Can you work these out from the model? Positions are in its coordinate system, mm. A direction names the side the tool comes from. Give positions to 0.01 mm unless a question says otherwise; leave off trailing zeros. Order: outer loops, then holes, each group sorted by start corner. A loop starts at its lowest first (then second) coordinate and runs counter-clockwise, first axis right, second up. Notation, with made-up numbers: (12, 10.5) -> (54, 10.5) arc R28 cw to (54, 36.5) -> close; hole circle Ø6 at (17, 40.25). An arc over 180 degrees is marked (long way). Answer as a JSON object with one key per item and string values.
Solid Edge part; units mm, degrees
sketch "Sketch1" plane through (0, 0, 0) normal (0, -1, 0) x (1, 0, 0)
  line L0 (0, 19.05) -> (0, 0)
  line L1 (0, 0) -> (19.05, 0)
  line L2 (19.05, 0) -> (19.05, 1.27)
  arc A0 (19.05, 1.27) -> (17.145, 3.175) centre (17.145, 1.27) ccw
  line L3 (17.145, 3.175) -> (6.985, 3.175)
  arc A1 (6.985, 3.175) -> (3.175, 6.985) centre (6.985, 6.985) cw
  line L4 (3.175, 6.985) -> (3.175, 17.145)
  arc A2 (3.175, 17.145) -> (1.27, 19.05) centre (1.27, 17.145) ccw
  line L5 (1.27, 19.05) -> (0, 19.05)
extrude "Protrusion1" add sketch "Sketch1" against normal blind 34.925
properties material "Steel"
1. Please list where these lines run through material, in increasing order: L1, parallel to Z at x = 13, y = 30 (3 decimals); L2, parallel to X at y = 23, z = 18.
Worked answers:
{"L1": "0 to 3.175", "L2": "0 to 2.97"}
2. For faces 1 (the face through (3.175, 17, 12)), 2 (the face through (9, 17, 0)), which set-ups out of +Z, -Z, +X, -X, +Y, -Y let a thin tool reach every point of the face, with its end or its side?
Worked answers:
{"face 1": "+Z, +X, +Y, -Y", "face 2": "-Z, +X, -X, +Y, -Y"}
3. If we section it at A-A on y = 29.5: Please give me the cut outline in (x, z) (3 decimals), then the cut area to 3 significant figures.
Worked answers:
{"outline": "(0, 0) -> (19.05, 0) -> (19.05, 1.27) arc R1.905 ccw to (17.145, 3.175) -> (6.985, 3.175) arc R3.81 cw to (3.175, 6.985) -> (3.175, 17.145) arc R1.905 ccw to (1.27, 19.05) -> (0, 19.05) -> close", "area": "112 mm²"}
4. If we section it at C-C on x = 10: Please give me the cut outline in (y, z) (3 decimals), then the cut area to 3 significant figures.
Worked answers:
{"outline": "(0, 0) -> (34.925, 0) -> (34.925, 3.175) -> (0, 3.175) -> close", "area": "111 mm²"}
5. If we section it at B-B on z = 15.25: Please give me the cut outline in (x, y) (3 decimals), then the cut area to 3 significant figures.
Worked answers:
{"outline": "(0, 0) -> (3.175, 0) -> (3.175, 34.925) -> (0, 34.925) -> close", "area": "111 mm²"}
6. Will these pins go through, and if not, where does the flat tip stop? pin 1 Ø5 at (y, z) = (25.5, 7.5) entering from +X; pin 2 Ø1.5 at (y, z) = (10.5, 15.5) entering from +X (3 decimals); pin 3 Ø8 at (x, y) = (9.5, 20.5) entering from +Z; pin 4 Ø6 at (x, y) = (16, 30) entering from -Z.
Worked answers:
{"pin 1": "x = 3.73", "pin 2": "x = 3.175", "pin 3": "z = 3.48", "pin 4": "z = 0"}
